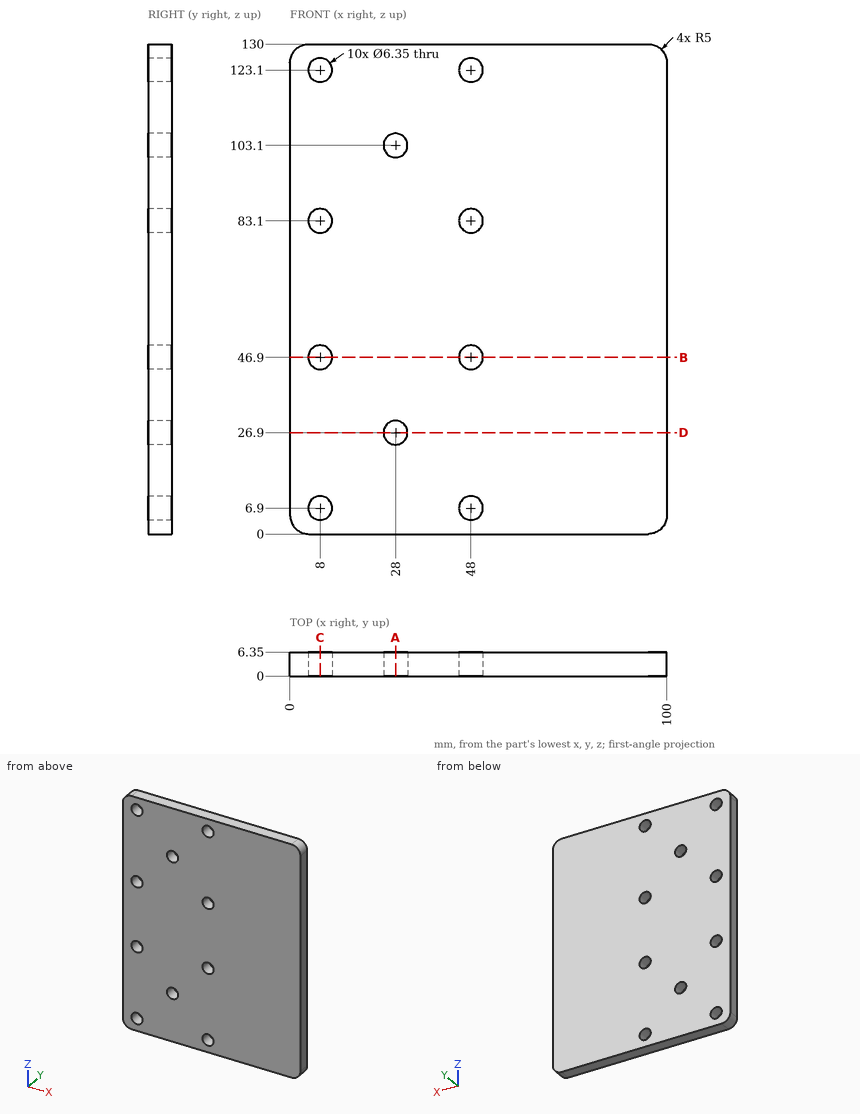
Study the drawing (mm; zero at the part's minimum x, y, z) and answer. Give positions to 0.01 mm unless a question says otherwise; leave off trailing zeros. Write each loop counter-clockwise with the first axis right and the second up, starting at its lowest first coordinate (ties: lowest second). Pieces come first, ordered by that corner, then holes. Notation, with made-up numbers: M -27,54.25 L -16,54.25 A24 ccw -16,75.25 Z; hole C 19.5,72.5 d10. An arc over 180 degrees is marked long. Put each result on its own line as item: value. Start each with the question number.
1. Consider line 1 along Z through (x, y) = (8, 4.75) (3 decimals); line 2 along X through (y, z) = (4.25, 123.1) (3 decimals); line 3 along Z through (x, y) = (28, 3.5) (3 decimals). Determine where each line is inside the solid, lowest interval first.
2. The part is cut by section C-C, the plane x = 8. Give the vertices of the cut face in (y, z) (3 decimals), and give its area (3 significant figures).
3. The part is cut by section B-B, the plane z = 46.9. Give the vertices of the cut face in (x, y) (3 decimals), and give its area (3 significant figures).
4. The part is cut by section D-D, the plane z = 26.9. Give the vertices of the cut face in (x, y) (3 decimals), and give its area (3 significant figures).
5. This flat-tipped pin is pushed along its axis until it touches: pin 1 Ø1 at (x, y) = (51.5, 2.5) entering from -Z. Where does it stop, or does it pass through?
6. The part is cut by section A-A, the plane x = 28. Give the vertices of the cut face in (y, z) (3 decimals), and give its area (3 significant figures).
Final values:
1. line 1: z = 0 to 3.725, 10.075 to 43.725, 50.075 to 79.925, 86.275 to 119.925, 126.275 to 130
1. line 2: x = 0 to 4.825, 11.175 to 44.825, 51.175 to 100
1. line 3: z = 0 to 23.725, 30.075 to 99.925, 106.275 to 130
2. outline: M 0,0 L 6.35,0 L 6.35,3.725 L 0,3.725 Z; M 0,10.075 L 6.35,10.075 L 6.35,43.725 L 0,43.725 Z; M 0,50.075 L 6.35,50.075 L 6.35,79.925 L 0,79.925 Z; M 0,86.275 L 6.35,86.275 L 6.35,119.925 L 0,119.925 Z; M 0,126.275 L 6.35,126.275 L 6.35,130 L 0,130 Z
2. area: 664 mm²
3. outline: M 0,0 L 4.825,0 L 4.825,6.35 L 0,6.35 Z; M 11.175,0 L 44.825,0 L 44.825,6.35 L 11.175,6.35 Z; M 51.175,0 L 100,0 L 100,6.35 L 51.175,6.35 Z
3. area: 554 mm²
4. outline: M 0,0 L 24.825,0 L 24.825,6.35 L 0,6.35 Z; M 31.175,0 L 100,0 L 100,6.35 L 31.175,6.35 Z
4. area: 595 mm²
5. pin 1: stops at z = 0
6. outline: M 0,0 L 6.35,0 L 6.35,23.725 L 0,23.725 Z; M 0,30.075 L 6.35,30.075 L 6.35,99.925 L 0,99.925 Z; M 0,106.275 L 6.35,106.275 L 6.35,130 L 0,130 Z
6. area: 745 mm²
